```python
from build123d import *

# Parameters (mm, degrees)
CORTAR_EXTRUIR1_REACH = 37.16
CROQUIS2_R            = 4
CROQUIS3_R            = 5
CORTAR_EXTRUIR2_DEPTH = 5


with BuildPart() as part:
    # Croquis1 → Revolución1 (revolve)
    with BuildSketch(Plane.XY):
        Polygon((0, 6), (0, -6), (-5.142300877, -12.128355545), (-5.142300877, -15.128355545), (4.857699123, -15.128355545), (4.857699123, 15.128355545), (-5.142300877, 15.128355545), (-5.142300877, 12.128355545), align=None)
    revolve(axis=Axis((4.857699123, 15.128355545, 0), (0, -1, 0)))

    # Croquis2 → Cortar-Extruir1 (cut, up to next)
    with BuildSketch(Plane.XZ.offset(15.128355545), mode=Mode.PRIVATE) as cortar_extruir1_sk1:
        with Locations((4.857699123, 0)):
            Circle(CROQUIS2_R)
    cortar_extruir1_tool1 = extrude(cortar_extruir1_sk1.sketch, amount=-CORTAR_EXTRUIR1_REACH, mode=Mode.PRIVATE) & part.part
    add(cortar_extruir1_tool1.solids().sort_by_distance((4.857699, -15.128356, 0))[0], mode=Mode.SUBTRACT)

    # Croquis3 → Cortar-Extruir2 (cut)
    with BuildSketch(Plane.XZ.offset(15.128355545)):
        with Locations((4.857699123, 0)):
            Circle(CROQUIS3_R)
    extrude(amount=-CORTAR_EXTRUIR2_DEPTH, mode=Mode.SUBTRACT)


solid = part.part
```
CAD build for the part. Positions are in the model's coordinates, mm. A direction names the side the tool comes from. Round coordinates to 2 decimals unless told otherwise and drop trailing zeros. Order: outer loops, then holes, each group sorted by start corner. A loop starts at its lowest first (then second) coordinate and runs counter-clockwise, first axis right, second up.
Item 1: Probe line 1 along Y through (x, z) = (6.75, 4); line 2 along Y through (x, z) = (-0.75, 5.5); line 3 along X through (y, z) = (5, -2). List the from-to ranges inside material, lowest first.
Item 2: Pin check, flat tips, straight feed: pin 1 (2 mm diameter, centred on x = 2, z = 0, fed in from +Y); pin 2 (4 mm diameter, centred on y = 10.5, z = 6.5, fed in from -X); pin 3 (5 mm diameter, centred on x = 11.5, y = -2.5, fed in from +Z); pin 4 (11 mm diameter, centred on x = 2.5, z = 0.5, fed in from -Y). Stop position of each tip, or through.
Item 3: Saw through at C-C on y = -8.5. Write the cut outline in (x, z), then the cut area to 3 significant figures.
Item 4: Saw through at B-B on y = -3.5. Write the cut outline in (x, z), then the cut area to 3 significant figures.
Item 5: Saw through at A-A on z = 0. Write the cut outline in (x, y).
Item 6: Tool access for faces 5 (the face through (9.627, -12.663, 1.502)), 6 (the face through (-4.68, 13.61, -3)), 7 (the face through (5.98, -6.383, 5.056)): list every direction of +Z, -Z, +X, -X, +Y, -Y with a clear straight run to the whole face (end or side of a thin tool).
Item 7: Mould opens along Y. For faces 1 (the face through (5.911, -0.084, 4.742)), 2 (the face through (9.2, 15.128, -0.1)), 3 (the face through (2.5, 6.3, 4.53)), 4 (the face through (-4.68, -13.65, -3)) say: pulls with the +Y half, pulls with the -Y half, needs draft (parallel to the pull), parting line crosses it, or undercut.
Reported:
1. line 1: y = -10.13 to 15.13
1. line 2: y = -15.13 to -9.57, 9.57 to 15.13
1. line 3: x = 0.43 to 1.39, 8.32 to 9.28
2. pin 1: passes through
2. pin 2: stops at x = -3.6
2. pin 3: stops at z = 2.54
2. pin 4: stops at y = -15.13
3. outline: circle Ø13.91 at (4.86, 0); hole circle Ø8 at (4.86, 0)
3. area: 102 mm2
4. outline: circle Ø9.72 at (4.86, 0); hole circle Ø8 at (4.86, 0)
4. area: 23.9 mm2
5. outline: (-5.14, -15.13) - (-0.14, -15.13) - (-0.14, -10.13) - (0.86, -10.13) - (0.86, 15.13) - (-5.14, 15.13) - (-5.14, 12.13) - (0, 6) - (0, -6) - (-5.14, -12.13) - close; (8.86, -10.13) - (9.86, -10.13) - (9.86, -15.13) - (14.86, -15.13) - (14.86, -12.13) - (9.72, -6) - (9.72, 6) - (14.86, 12.13) - (14.86, 15.13) - (8.86, 15.13) - close
6. face 5: -Y
6. face 6: +Y, -Y
6. face 7: none
7. face 1: undercut
7. face 2: pulls with the +Y half
7. face 3: undercut
7. face 4: needs draft
